CAD build for the part. Positions are in the model's coordinates, mm. Coordinates: 2 decimals unless noted, no trailing zeros. Loops run counter-clockwise (first coordinate to the right, second up) from the corner with the lowest first, then second, coordinate; pieces in that order, holes last. Notation, with made-up numbers: (1, 70) -> (41, 70) arc R14 cw to (41, 77) -> close; hole circle Ø9 at (17.25, -36). An arc over 180 degrees is marked (long way). Return JSON: item names as keys, results as strings. Group by question number.
(1) Probe L1, parallel to X at y = 1.4, z = 3; L2, parallel to X at y = 0.5, z = 13; L3, parallel to Z at x = 69.5, y = -0.4. List the from-to ranges inside material, lowest first.
(2) Saw through at A-A on z = -2.5. Write the cut outline in (x, y).
(3) Saw through at B-B on y = 0. Write the cut outline in (x, z), then the cut area to 3 significant figures.
(4) Saw through at D-D on x = 40. Write the cut outline in (y, z).
(5) Flat gauge pins, fed straight in: pin 1 Ø1.2 at (x, y) = (77.5, -0.5) entering from +Z; pin 2 Ø1.2 at (x, y) = (43, 1) entering from -Z; pin 3 Ø2 at (x, y) = (46.5, -0.5) entering from +Z. Where does each tip first touch, or does it go through?
(6) Saw through at C-C on z = 21.5. Write the cut outline in (x, y).
```python
from build123d import *

# Parameters (mm, degrees)
EXTRUDE_1_DEPTH     = 80
SKETCH_3_W          = 60
SKETCH_3_H          = 16.054950693
SKETCH_3_H_2        = 56.960343262
CUT_EXTRUDE_1_DEPTH = 10
SKETCH_4_W          = 5
SKETCH_4_H          = 20
CUT_EXTRUDE_2_DEPTH = 10


with BuildPart() as part:
    # 草图2 → 凸台-拉伸1 (new body)
    with BuildSketch(Plane(origin=(0, 0, 0), x_dir=(0, 0, -1), z_dir=(1, 0, 0))):
        with BuildLine():
            Line((-28, 2), (28, 2))
            ThreePointArc((28, 2), (30, 0), (28, -2))
            Line((28, -2), (-28, -2))
            ThreePointArc((-28, -2), (-30, 0), (-28, 2))
        make_face()
    extrude(amount=EXTRUDE_1_DEPTH)

    # 草图3 → 切除-拉伸1 (cut)
    with BuildSketch(Plane(origin=(0, 2, 0), x_dir=(1, 0, 0), z_dir=(0, 1, 0))):
        with Locations((40, -32.027475346)):
            Rectangle(SKETCH_3_W, SKETCH_3_H)
        with Locations((40, 8.480171631)):
            Rectangle(SKETCH_3_W, SKETCH_3_H_2)
    extrude(amount=-CUT_EXTRUDE_1_DEPTH, mode=Mode.SUBTRACT)

    # 草图4 → 切除-拉伸2 (cut)
    with BuildSketch(Plane(origin=(0, 2, 0), x_dir=(1, 0, 0), z_dir=(0, 1, 0))):
        with Locations((2.5, -20)):
            Rectangle(SKETCH_4_W, SKETCH_4_H)
        with Locations((77.5, -20)):
            Rectangle(SKETCH_4_W, SKETCH_4_H)
    extrude(amount=-CUT_EXTRUDE_2_DEPTH, mode=Mode.SUBTRACT)


solid = part.part
```
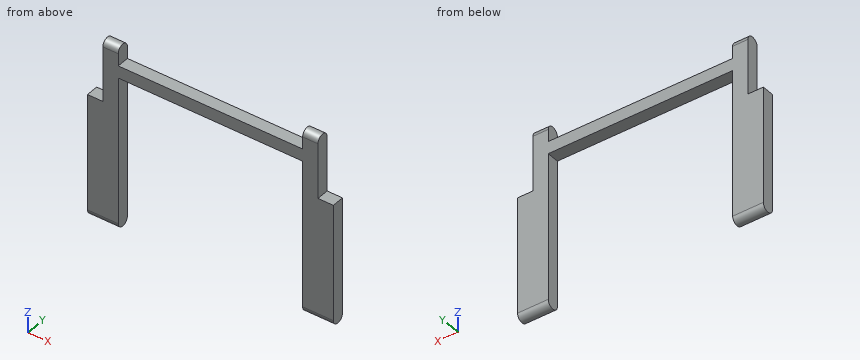
Geometry results:
{
 "1": {"L1": "0 to 10, 70 to 80", "L2": "5 to 10, 70 to 75", "L3": "20 to 24"},
 "2": {"outline": "(0, -2) -> (10, -2) -> (10, 2) -> (0, 2) -> close; (70, -2) -> (80, -2) -> (80, 2) -> (70, 2) -> close"},
 "3": {"outline": "(0, -30) -> (10, -30) -> (10, 20) -> (70, 20) -> (70, -30) -> (80, -30) -> (80, 10) -> (75, 10) -> (75, 30) -> (70, 30) -> (70, 24) -> (10, 24) -> (10, 30) -> (5, 30) -> (5, 10) -> (0, 10) -> close", "area": "1,240 mm²"},
 "4": {"outline": "(-2, 20) -> (2, 20) -> (2, 24) -> (-2, 24) -> close"},
 "5": {"pin 1": "z = 10", "pin 2": "z = 20", "pin 3": "z = 24"},
 "6": {"outline": "(5, -2) -> (75, -2) -> (75, 2) -> (5, 2) -> close"}
}
